```python
from build123d import *

# Parameters (mm, degrees)
BOSS_EXTRU_1_DEPTH      = 15
ESQUISSE2_R             = 2
ENL_V_MAT_EXTRU_1_DEPTH = 12
ESQUISSE3_R             = 2
ENL_V_MAT_EXTRU_2_DEPTH = 12
CONG_1_R                = 1
ENL_V_MAT_EXTRU_3_REACH = 28.101


with BuildPart() as part:
    # Esquisse1 → Boss.-Extru.1 (new body)
    with BuildSketch(Plane(origin=(0, 0, 0), x_dir=(1, 0, 0), z_dir=(0, 1, 0))):
        Polygon((0, 0), (7.5, 0), (7.5, 20), (-7.5, 20), (-7.5, 0), align=None)
    extrude(amount=BOSS_EXTRU_1_DEPTH)

    # Esquisse2 → Enlèv. mat.-Extru.1 (cut)
    with BuildSketch(Plane.XZ):
        with Locations(Location((-3, -16, 0), (0, 0, 270))):
            Circle(ESQUISSE2_R)
        with Locations(Location((3, -4, 0), (0, 0, 270))):
            Circle(ESQUISSE2_R)
    extrude(amount=-ENL_V_MAT_EXTRU_1_DEPTH, mode=Mode.SUBTRACT)

    # Esquisse3 → Enlèv. mat.-Extru.2 (cut)
    with BuildSketch(Plane.XY):
        with Locations((-3, 10)):
            Circle(ESQUISSE3_R)
    extrude(amount=-ENL_V_MAT_EXTRU_2_DEPTH, mode=Mode.SUBTRACT)

    # Congé1
    cong_1_edges = [part.edges().sort_by_distance(p)[0] for p in [
        (-7.5, 7.5, 0),
        (-7.5, 7.5, -20),
        (7.5, 7.5, -20),
    ]]
    fillet(cong_1_edges, radius=CONG_1_R)

    # Esquisse5 → Enlèv. mat.-Extru.3 (cut, up to next)
    with BuildSketch(Plane(origin=(0, 15, 0), x_dir=(1, 0, 0), z_dir=(0, 1, 0)), mode=Mode.PRIVATE) as enl_v_mat_extru_3_sk1:
        Polygon((7.5, 0), (2.3, 0), (7.5, 1.5), align=None)
    enl_v_mat_extru_3_tool1 = extrude(enl_v_mat_extru_3_sk1.sketch, amount=-ENL_V_MAT_EXTRU_3_REACH, mode=Mode.PRIVATE) & part.part
    add(enl_v_mat_extru_3_tool1.solids().sort_by_distance((5.766667, 15, -0.5))[0], mode=Mode.SUBTRACT)


solid = part.part
```
Geometry check sheet. Reference: the model listing, model coordinates, mm. A direction names the side the tool comes from. Round coordinates to 2 decimals unless told otherwise and drop trailing zeros. Loops run counter-clockwise (first coordinate to the right, second up) from the corner with the lowest first, then second, coordinate; pieces in that order, holes last. Notation, with made-up numbers: (36, 84.25) - (84, 84.25) arc R29 ccw to (84, 121.25) - close; hole circle Ø2 at (-5.5, 68.25). An arc over 180 degrees is marked (long way). Write each question's results on one line, items separated by ' | '. Start each with the question number.
Q1. Gauge pin test, flat ends, axial feed: P1, Ø2, axis at x = 5, y = 4, coming from the +Z side; P2, Ø1.2, axis at x = 2.5, z = -4, coming from the -Y side; P3, Ø5, axis at x = 2, y = 6, coming from the +Z side; P4, Ø2, axis at x = -3.5, y = 9.5, coming from the +Z side. Record the tip position at first contact, or that the pin passes through.
Q2. Release check for a two-part mould opening along X. For faces 4 (the flat face through (0, 7, -20)), 5 (the flat face through (3, 12, -4)), 6 (the flat face through (4.86, 7.6, -0.74)) record: +X half, -X half, draft (parallel to the pull), parting line (faces both ways), or undercut.
Q3. Cross-section at C-C on z = -16. Enter the section's corners in (x, y), and give its area (3 significant figures).
Q4. Thickness scan on line 1 (Y direction, x = -3, z = -8.5); line 2 (X direction, y = 9, z = -16); line 3 (X direction, y = 5.5, z = -4). Record the ranges inside material, lowest first. Write a range as [from, to].
Q5. Cross-section at D-D on x = -3. Enter the section's corners in (y, z).
Q6. Access from +Z, -Z, +X, -X, +Y, -Y to the whole of each face (thin tool, end or side, straight path). Record for faces 1 (the cylindrical face through (-3, 12, -6)), 2 (the flat face through (-3, 12, -16)), 3 (the flat face through (0, 0, -10)).
Q7. Cross-section at B-B on z = -10.25. Enter the section's corners in (x, y), and give its area (3 significant figures).
Q8. Cross-section at A-A on y = 4. Enter the section's corners in (x, z).
Answers below:
1) P1: stops at z = -0.49 | P2: stops at y = 12 | P3: stops at z = 0 | P4: stops at z = -12
2) face 4: draft | face 5: undercut | face 6: +X half
3) outline: (-7.5, 0) - (-5, 0) - (-5, 12) - (-1, 12) - (-1, 0) - (7.5, 0) - (7.5, 15) - (-7.5, 15) - close | area: 177 mm²
4) line 1: y = [0, 8], [12, 15] | line 2: x = [-7.5, -5], [-1, 7.5] | line 3: x = [-7.5, 1], [5, 7.5]
5) outline: (0, -20) - (15, -20) - (15, 0) - (12, 0) - (12, -12) - (8, -12) - (8, 0) - (0, 0) - (0, -14) - (12, -14) - (12, -18) - (0, -18) - close
6) face 1: +Z | face 2: -Y | face 3: +Z, -Z, +X, -X, -Y
7) outline: (-7.5, 0) - (7.5, 0) - (7.5, 15) - (-7.5, 15) - close; hole circle Ø4 at (-3, 10) | area: 212 mm²
8) outline: (-7.5, -19) arc R1 ccw to (-6.5, -20) - (6.5, -20) arc R1 ccw to (7.5, -19) - (7.5, -1.5) - (2.3, 0) - (-6.5, 0) arc R1 ccw to (-7.5, -1) - close; hole circle Ø4 at (-3, -16); hole circle Ø4 at (3, -4)
